Check sheet for the modelled part. Datum: model origin and axes. Units: mm. Face numbers are marked on the shaded views. A direction names the side the tool comes from. Round coordinates to 2 decimals unless told otherwise and drop trailing zeros. Order: outer loops, then holes, each group sorted by start corner. A loop starts at its lowest first (then second) coordinate and runs counter-clockwise, first axis right, second up. Notation, with made-up numbers: (38.5, 28) -> (69.5, 28) arc R13 cw to (69.5, 41) -> close; hole circle Ø1 at (75.25, 26.25). An arc over 180 degrees is marked (long way). Answer in a Markdown table with one row per item.
from build123d import *

# Parameters (mm, degrees)
ESBO_O1_R                = 11.5
RESSALTO_EXTRUS_O1_DEPTH = 17.5
FILLET1_R                = 5
ESBO_O2_R                = 2
CORTE_EXTRUS_O1_DEPTH    = 10


with BuildPart() as part:
    # Esboço1 → Ressalto-extrusão1 (new, symmetric)
    with BuildSketch(Plane(origin=(0, 0, 0), x_dir=(0, 0, -1), z_dir=(1, 0, 0))):
        with BuildLine():
            Line((-9.301463672, 35.294939773), (-15.923932545, 48.753873832))
            ThreePointArc((-15.923932545, 48.753873832), (-31.882117783, 25.625328571), (-36.439403175, -2.102354921))
            ThreePointArc((-36.439403175, -2.102354921), (29.541430866, -21.43720743), (-9.301463672, 35.294939773))
        make_face()
        Circle(ESBO_O1_R, mode=Mode.SUBTRACT)
        with BuildLine():
            ThreePointArc((-30.461709826, 5.751889646), (-17.884176458, 25.321063019), (4.764081686, 30.631740494))
            ThreePointArc((4.764081686, 30.631740494), (8.936284719, 24.922736917), (3.227281142, 20.750533883))
            ThreePointArc((3.227281142, 20.750533883), (-12.115087278, 17.152978174), (-20.635351817, 3.896441373))
            ThreePointArc((-20.635351817, 3.896441373), (-26.476254958, -0.089013495), (-30.461709826, 5.751889646))
        make_face(mode=Mode.SUBTRACT)
    extrude(amount=RESSALTO_EXTRUS_O1_DEPTH, both=True)

    # Fillet1
    fillet1_edges = [part.edges().sort_by_distance(p)[0] for p in [
        (0, 35.294939773, 9.301463672),
    ]]
    fillet(fillet1_edges, radius=FILLET1_R)

    # Esboço2 → Corte-extrusão1 (cut)
    with BuildSketch(Plane(origin=(17.5, 0, 0), x_dir=(0, 0, -1), z_dir=(1, 0, 0))):
        with Locations((-9.374769917, 13.273137873)):
            Circle(ESBO_O2_R)
        with Locations((13.273137873, 9.374769917)):
            Circle(ESBO_O2_R)
        with Locations((9.374769917, -13.273137873)):
            Circle(ESBO_O2_R)
        with Locations((-13.273137873, -9.374769917)):
            Circle(ESBO_O2_R)
    extrude(amount=-CORTE_EXTRUS_O1_DEPTH, mode=Mode.SUBTRACT)


solid = part.part
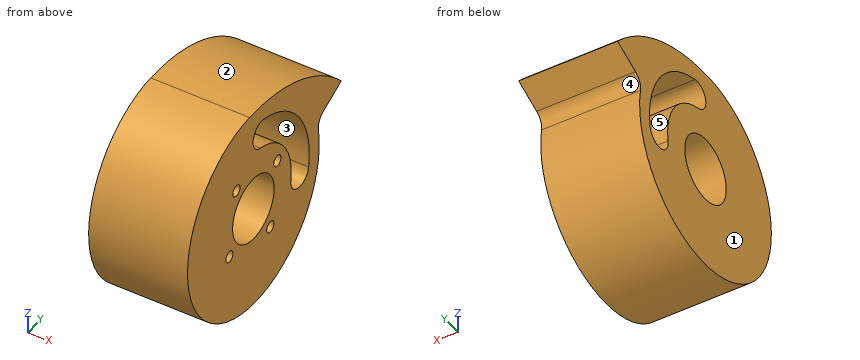
Item 1: Mould release check, pull along Z, two halves, no side actions. Record for the marked faces 1, 2 and 3: pulls with the +Z half, pulls with the -Z half, needs draft (parallel to the pull), parting line crosses it, or undercut.
Result sheet:
| item | result |
|---|---|
| face 1 | needs draft |
| face 2 | pulls with the +Z half |
| face 3 | undercut |
Item 2: Depth check by flat-ended pin: P1, Ø8, axis at x = -10.5, z = 9.5, coming from the +Y side; P2, Ø8, axis at x = -14, y = -22, coming from the -Z side; P3, Ø6, axis at x = 1.5, z = 25, coming from the -Y side; P4, Ø14, axis at y = 0, z = 0, coming from the -X side. Enter the tip coordinate at first touch or a pass-through.
Result sheet:
| item | result |
|---|---|
| P1 | stops at y = 43.83 |
| P2 | stops at z = -31.75 |
| P3 | stops at y = -29.12 |
| P4 | passes through |
Item 3: Scan lines: line 1 (Y direction, x = -5.5, z = 0); line 2 (Y direction, x = -5.5, z = 16); line 3 (Y direction, x = 8.5, z = 27.5). Record each from-to range of solid material in increasing order. Write a range as [from, to].
Result sheet:
| item | result |
|---|---|
| line 1 | y = [-36.5, -11.5], [11.5, 21], [31, 36.5] |
| line 2 | y = [-32.81, 13.6], [26.55, 48.68] |
| line 3 | y = [-24, 0.22], [14.31, 34.46] |
Item 4: Cross-section at A-A (z = 0). Record the boundary of the cut face in (x, y), and give its area (3 significant figures).
Result sheet:
| item | result |
|---|---|
| outline | (-17.5, -36.5) -> (17.5, -36.5) -> (17.5, -11.5) -> (-17.5, -11.5) -> close; (-17.5, 11.5) -> (17.5, 11.5) -> (17.5, 21) -> (-17.5, 21) -> close; (-17.5, 31) -> (17.5, 31) -> (17.5, 36.5) -> (-17.5, 36.5) -> close |
| area | 1,400 mm^2 |
Item 5: Cross-section at B-B (x = 10). Record the boundary of the cut face in (y, z).
Result sheet:
| item | result |
|---|---|
| outline | (-2.1, 36.44) arc R36.5 ccw (long way) to (36.05, 5.74) arc R5 cw to (38.78, 11.01) -> (48.75, 15.92) arc R64.23 ccw to start; hole circle Ø4 at (-13.27, -9.37); hole circle Ø23 at (0, 0); hole circle Ø4 at (-9.37, 13.27); hole (3.9, 20.64) arc R21 cw to (20.75, -3.23) arc R5 ccw to (30.63, -4.76) arc R31 ccw to (5.75, 30.46) arc R5 ccw to start; hole circle Ø4 at (9.37, -13.27); hole circle Ø4 at (13.27, 9.37) |
Item 6: Cross-section at D-D (y = 27). Record the boundary of the cut face in (x, z), and give its area (3 significant figures).
Result sheet:
| item | result |
|---|---|
| outline | (-17.5, -24.56) -> (17.5, -24.56) -> (17.5, -8.82) -> (-17.5, -8.82) -> close; (-17.5, 15.23) -> (17.5, 15.23) -> (17.5, 31.31) -> (-17.5, 31.31) -> close |
| area | 1,110 mm^2 |
Item 7: Cross-section at C-C (y = 2). Record the boundary of the cut face in (x, z).
Result sheet:
| item | result |
|---|---|
| outline | (-17.5, -36.45) -> (17.5, -36.45) -> (17.5, -11.32) -> (-17.5, -11.32) -> close; (-17.5, 11.32) -> (17.5, 11.32) -> (17.5, 21.42) -> (-17.5, 21.42) -> close; (-17.5, 29.67) -> (17.5, 29.67) -> (17.5, 36.54) -> (-17.5, 36.54) -> close |
Item 8: Set-up check for the marked faces 4 and 5: record each of +Z, -Z, +X, -X, +Y, -Y from which the full face is reachable in a straight line by a thin tool's end or side.
Result sheet:
| item | result |
|---|---|
| face 4 | +X, -X, +Y |
| face 5 | +X, -X |
